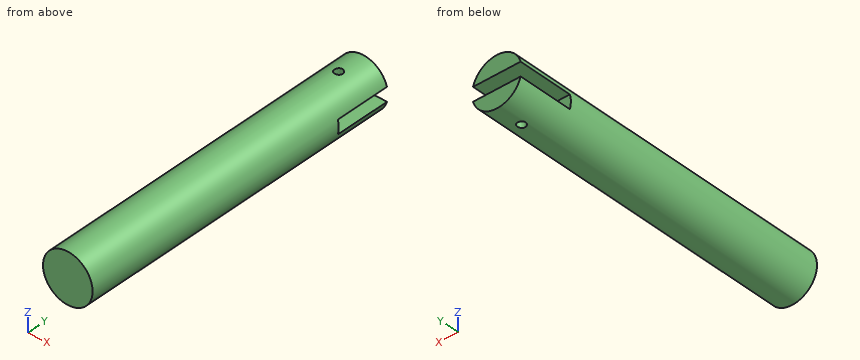
from build123d import *

# Parameters (mm, degrees)
SKETCH1_R               = 18
BOSS_EXTRUDE1_DEPTH     = 120
SKETCH2_W               = 50
SKETCH2_H               = 10
CUT_EXTRUDE1_DEPTH      = 40
CUT_EXTRUDE2_DEPTH      = 123.670289802
CUT_EXTRUDE2_DEPTH_BACK = 123.670289802
SKETCH3_R               = 3


with BuildPart() as part:
    # Sketch1 → Boss-Extrude1 (new, symmetric)
    with BuildSketch(Plane(origin=(0, 0, 0), x_dir=(1, 0, 0), z_dir=(0, 1, 0))):
        with Locations(Location((0, 0, 0), (0, 0, 270))):
            Circle(SKETCH1_R)
    extrude(amount=BOSS_EXTRUDE1_DEPTH, both=True)

    # Sketch2 → Cut-Extrude1 (cut)
    with BuildSketch(Plane(origin=(0, 120, 0), x_dir=(1, 0, 0), z_dir=(0, 1, 0))):
        Rectangle(SKETCH2_W, SKETCH2_H)
    extrude(amount=-CUT_EXTRUDE1_DEPTH, mode=Mode.SUBTRACT)

    # Sketch3 → Cut-Extrude2 (cut, two sides: drawn at the far end of the back side and taken through both)
    with BuildSketch(Plane.XY.offset(-CUT_EXTRUDE2_DEPTH_BACK)):
        with Locations(Location((0, 100, 0), (0, 0, 90))):
            Circle(SKETCH3_R)
    extrude(amount=CUT_EXTRUDE2_DEPTH + CUT_EXTRUDE2_DEPTH_BACK, mode=Mode.SUBTRACT)


solid = part.part
Read the model definition and answer for the solid it produces. Units are mm, in the model's axes. Give positions to 0.01 mm unless a question says otherwise; leave off trailing zeros. Write each loop counter-clockwise with the first axis right and the second up, starting at its lowest first coordinate (ties: lowest second). Pieces come first, ordered by that corner, then holes. Notation, with made-up numbers: (67.5, 3) -> (96.5, 3) arc R31 ccw to (96.5, 29) -> close; hole circle Ø1 at (50, 14). An arc over 180 degrees is marked (long way). Answer as a JSON object with one key per item and string values. Group by question number.
1) Each of these flat-tipped pins is pushed along its axis until it touches: P1, Ø4, axis at x = -14, y = -53, coming from the -Z side; P2, Ø3, axis at y = -95, z = -9.5, coming from the -X side; P3, Ø12, axis at y = -18, z = 12, coming from the -X side. Where does it stop, or does it pass through?
2) Find section C-C (z = -10). Write down the section's boundary in (x, y).
3) Find section D-D (x = 15). Write down the section's boundary in (y, z), and give its area (3 significant figures).
4) Find section B-B (x = 0). Write down the section's boundary in (y, z), and give its area (3 significant figures).
5) Find section A-A (y = 99.5). Write down the section's boundary in (x, z), and give its area (3 significant figures).
6) Consider L1, parallel to Y at x = 0, z = 8; L2, parallel to Z at x = -5, y = 104.5; L3, parallel to X at y = 100, z = 11. Determine where each line is inside the solid, lowest interval first. Write a range as from..to.
Values follow:
{
 "1": {"P1": "stops at z = -13.42", "P2": "stops at x = -16.12", "P3": "stops at x = -16.97"},
 "2": {"outline": "(-14.97, -120) -> (14.97, -120) -> (14.97, 120) -> (-14.97, 120) -> close; hole circle Ø6 at (0, 100)"},
 "3": {"outline": "(-120, -9.95) -> (120, -9.95) -> (120, -5) -> (80, -5) -> (80, 5) -> (120, 5) -> (120, 9.95) -> (-120, 9.95) -> close", "area": "4,380 mm2"},
 "4": {"outline": "(-120, -18) -> (97, -18) -> (97, -5) -> (80, -5) -> (80, 5) -> (97, 5) -> (97, 18) -> (-120, 18) -> close; (103, -18) -> (120, -18) -> (120, -5) -> (103, -5) -> close; (103, 5) -> (120, 5) -> (120, 18) -> (103, 18) -> close", "area": "8,080 mm2"},
 "5": {"outline": "(-17.29, -5) arc R18 ccw to (-2.96, -17.76) -> (-2.96, -5) -> close; (-17.29, 5) -> (-2.96, 5) -> (-2.96, 17.76) arc R18 ccw to start; (2.96, -17.76) arc R18 ccw to (17.29, -5) -> (2.96, -5) -> close; (2.96, 5) -> (17.29, 5) arc R18 ccw to (2.96, 17.76) -> close", "area": "510 mm2"},
 "6": {"L1": "y = -120..97, 103..120", "L2": "z = -17.29..-5, 5..17.29", "L3": "x = -14.25..-3, 3..14.25"}
}
